Source: three-view drawing plus pictorial views. Frame: mm from the lowest corner of the part. A direction names the side the tool comes from. Give positions to 0.01 mm unless a question says otherwise; leave off trailing zeros. Order: outer loops, then holes, each group sorted by start corner. A loop starts at its lowest first (then second) coordinate and runs counter-clockwise, first axis right, second up.
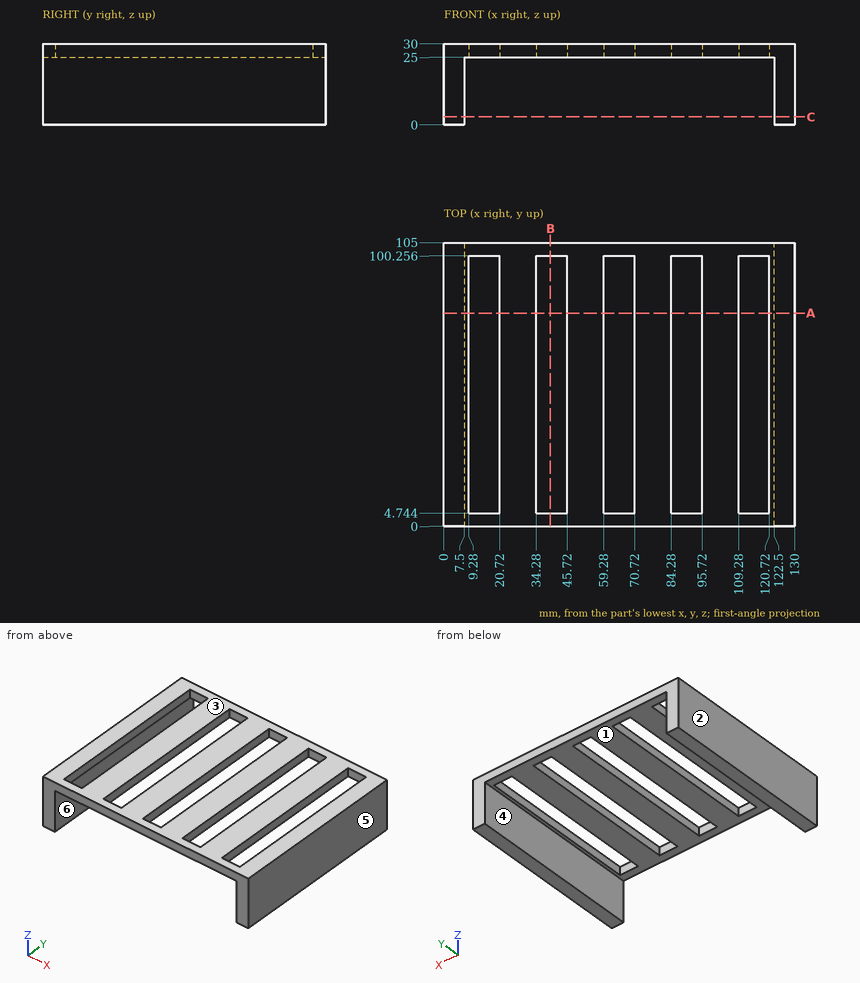
1) Section query B-B on x = 39.5. Output: boundary loops of the cut face in (y, z).
Checks:
outline: (0, 25) - (4.74, 25) - (4.74, 30) - (0, 30) - close; (100.26, 25) - (105, 25) - (105, 30) - (100.26, 30) - close
2) Ray query, L1, parallel to X at y = 33, z = 25.75; L2, parallel to X at y = 64, z = 7; L3, parallel to Y at x = 43, z = 26.25. Return the intervals inside material, ascending.
Checks:
L1: x = 0 to 9.28, 20.72 to 34.28, 45.72 to 59.28, 70.72 to 84.28, 95.72 to 109.28, 120.72 to 130
L2: x = 0 to 7.5, 122.5 to 130
L3: y = 0 to 4.74, 100.26 to 105
3) Reachability of the marked faces 1 and 2 from +Z, -Z, +X, -X, +Y, -Y: full face, straight path, thin tool, end or side. Return the list, or none.
Checks:
face 1: -Z, +Y, -Y
face 2: +Z, -Z, -X, +Y, -Y
4) Pull-direction query (X, two-part tool) for the marked faces 3, 4, 5 and 6; classes: +X half, -X half, draft (parallel to the pull), parting line (faces both ways), or undercut.
Checks:
face 3: draft
face 4: undercut
face 5: +X half
face 6: undercut
5) Section query C-C on z = 3. Output: boundary loops of the cut face in (x, y), and give its area (4 significant figures).
Checks:
outline: (0, 0) - (7.5, 0) - (7.5, 105) - (0, 105) - close; (122.5, 0) - (130, 0) - (130, 105) - (122.5, 105) - close
area: 1,575 mm2
6) First-contact query: pin 1 Ø4 at (x, y) = (101, 22.5) entering from -Z. Flat tip, straight axial feed; report the tip coordinate or a pass-through.
Checks:
pin 1: stops at z = 25
7) Section query A-A on y = 79. Output: boundary loops of the cut face in (x, z).
Checks:
outline: (0, 0) - (7.5, 0) - (7.5, 25) - (9.28, 25) - (9.28, 30) - (0, 30) - close; (20.72, 25) - (34.28, 25) - (34.28, 30) - (20.72, 30) - close; (45.72, 25) - (59.28, 25) - (59.28, 30) - (45.72, 30) - close; (70.72, 25) - (84.28, 25) - (84.28, 30) - (70.72, 30) - close; (95.72, 25) - (109.28, 25) - (109.28, 30) - (95.72, 30) - close; (120.72, 25) - (122.5, 25) - (122.5, 0) - (130, 0) - (130, 30) - (120.72, 30) - close
